```python
from build123d import *

# Parameters (mm, degrees)
F0_R     = 30
F0_R_2   = 2.9
F0_R_3   = 11.5
F1_DEPTH = 6.2
F2_SIZE  = 5


with BuildPart() as f1:
    # F0 (on Top) → F1 (new body)
    with BuildSketch(Plane.XY):
        Circle(F0_R)
        with Locations((0, -17)):
            Circle(F0_R_2, mode=Mode.SUBTRACT)
        Circle(F0_R_3, mode=Mode.SUBTRACT)
        with Locations((0, 17)):
            Circle(F0_R_2, mode=Mode.SUBTRACT)
    extrude(amount=F1_DEPTH)

    # F2
    f2_edges = [f1.edges().sort_by_distance(p)[0] for p in [
        (-30, 0, 6.2),
    ]]
    chamfer(f2_edges, length=F2_SIZE)


solid = f1.part
```
Input: part model. Units: mm. Frame: model coordinates. Round coordinates to 2 decimals unless told otherwise and drop trailing zeros. Write each loop counter-clockwise with the first axis right and the second up, starting at its lowest first coordinate (ties: lowest second). Pieces come first, ordered by that corner, then holes. Notation, with made-up numbers: (88, 5.5) - (107, 5.5) arc R26 ccw to (107, 32.5) - close; hole circle Ø4 at (-25.75, 44.25). An arc over 180 degrees is marked (long way). Write item = value, one per line.
(1) Contact query for flat-ended pins moving along their axis: pin 1 Ø10 at (x, y) = (4, -10.5) entering from -Z; pin 2 Ø1 at (x, y) = (10, 1.5) entering from +Z; pin 3 Ø2 at (x, z) = (10, 2) entering from +Y; pin 4 Ø1 at (y, z) = (18.5, 4.5) entering from +X. Output: stop coordinate, or through.
Geometry check:
pin_1 = 0
pin_2 = through
pin_3 = 28.49
pin_4 = 20.08
(2) Section query B-B on x = 0. Output: boundary loops of the cut face in (y, z).
Geometry check:
outline = (-30, 0) - (-19.9, 0) - (-19.9, 6.2) - (-25, 6.2) - (-30, 1.2) - close; (-14.1, 0) - (-11.5, 0) - (-11.5, 6.2) - (-14.1, 6.2) - close; (11.5, 0) - (14.1, 0) - (14.1, 6.2) - (11.5, 6.2) - close; (19.9, 0) - (30, 0) - (30, 1.2) - (25, 6.2) - (19.9, 6.2) - close
(3) Section query C-C on z = 3.5. Output: boundary loops of the cut face in (x, y), then the cut area to 3 significant figures.
Geometry check:
outline = circle Ø55.4 at (0, 0); hole circle Ø23 at (0, 0); hole circle Ø5.8 at (0, -17); hole circle Ø5.8 at (0, 17)
area = 1,940 mm^2
(4) Section query A-A on y = 0. Output: boundary loops of the cut face in (x, z).
Geometry check:
outline = (-30, 0) - (-11.5, 0) - (-11.5, 6.2) - (-25, 6.2) - (-30, 1.2) - close; (11.5, 0) - (30, 0) - (30, 1.2) - (25, 6.2) - (11.5, 6.2) - close
(5) Pull-direction query (Y, two-part tool) for faces 1 (the conical face through (24.077, 7.582, 5.957)), 2 (the cylindrical face through (-1.5, 11.4, 3.1)), 3 (the flat face through (11, -5, 6.2)); classes: +Y half, -Y half, draft (parallel to the pull), parting line (faces both ways), or undercut.
Geometry check:
face_1 = parting line
face_2 = undercut
face_3 = draft
(6) Material intervals for probe 1 along Y at (x, z) = (0, 4.75); probe 2 along Y at (x, z) = (-5, 4); probe 3 along X at (y, z) = (-8.5, 1), sorted ascending.
Geometry check:
probe_1 = -26.45 to -19.9, -14.1 to -11.5, 11.5 to 14.1, 19.9 to 26.45
probe_2 = -26.74 to -10.36, 10.36 to 26.74
probe_3 = -28.77 to -7.75, 7.75 to 28.77
